Can you work these out from the model? Positions are in its coordinate system, mm. Face numbers are marked on the shaded views. A direction names the side the tool comes from. Give positions to 0.01 mm unless a question says otherwise; leave off trailing zeros. Order: outer loops, then holes, each group sorted by start corner. A loop starts at its lowest first (then second) coordinate and runs counter-clockwise, first axis right, second up. Notation, with made-up numbers: M -25.75,45.25 L -9.75,45.25 A16 cw -9.75,74.25 Z; hole C -21.5,-39 d7. An arc over 180 degrees is marked long. Write each question's results on one line, items separated by ' | '.
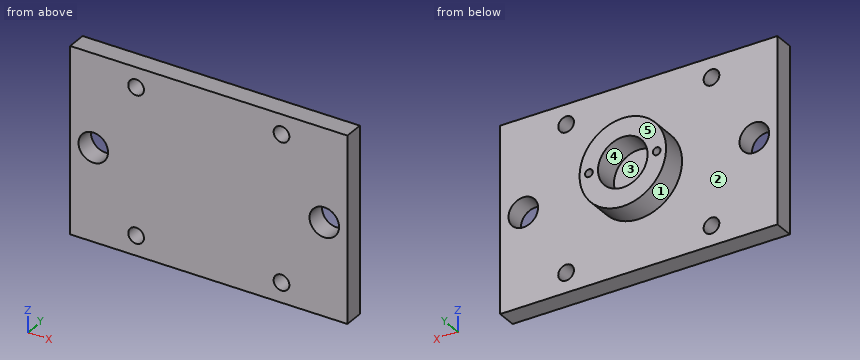
from build123d import *

# Parameters (mm, degrees)
SKETCH1_W           = 90
SKETCH1_H           = 60
SKETCH1_R           = 4.8
SKETCH1_R_2         = 2.55
BOSS_EXTRUDE1_DEPTH = 6.35
SKETCH2_R           = 14.05
SKETCH2_R_2         = 8.05
BOSS_EXTRUDE2_DEPTH = 8.175
SKETCH3_R           = 1.25
CUT_EXTRUDE1_DEPTH  = 8


with BuildPart() as part:
    # Sketch1 → Boss-Extrude1 (new body)
    with BuildSketch(Plane(origin=(0, 0, 0), x_dir=(1, 0, 0), z_dir=(0, 1, 0))):
        Rectangle(SKETCH1_W, SKETCH1_H)
        with Locations((-37.5, 0)):
            Circle(SKETCH1_R, mode=Mode.SUBTRACT)
        with Locations((37.5, 0)):
            Circle(SKETCH1_R, mode=Mode.SUBTRACT)
        with Locations((-23.6, -23.6)):
            Circle(SKETCH1_R_2, mode=Mode.SUBTRACT)
        with Locations((23.6, -23.6)):
            Circle(SKETCH1_R_2, mode=Mode.SUBTRACT)
        with Locations((23.6, 23.6)):
            Circle(SKETCH1_R_2, mode=Mode.SUBTRACT)
        with Locations((-23.6, 23.6)):
            Circle(SKETCH1_R_2, mode=Mode.SUBTRACT)
    extrude(amount=BOSS_EXTRUDE1_DEPTH)

    # Sketch2 → Boss-Extrude2 (add)
    with BuildSketch(Plane(origin=(0, 6.35, 0), x_dir=(1, 0, 0), z_dir=(0, 1, 0))):
        Circle(SKETCH2_R)
        Circle(SKETCH2_R_2, mode=Mode.SUBTRACT)
    extrude(amount=BOSS_EXTRUDE2_DEPTH)

    # Sketch3 → Cut-Extrude1 (cut)
    with BuildSketch(Plane(origin=(0, 14.525, 0), x_dir=(1, 0, 0), z_dir=(0, 1, 0))):
        with Locations((-11, 0)):
            Circle(SKETCH3_R)
        with Locations((11, 0)):
            Circle(SKETCH3_R)
    extrude(amount=-CUT_EXTRUDE1_DEPTH, mode=Mode.SUBTRACT)


solid = part.part
(1) We'd pull the mould along Z, two halves only. Please class the marked faces 1, 2 and 3: +Z half, -Z half, draft (parallel to the pull), parting line (faces both ways), or undercut.
Data:
face 1: parting line | face 2: draft | face 3: undercut
(2) Imagine slicing it at D-D, the plane x = -37.5. Write out the boundary of the cut face in (y, z), plus the area to 3 significant figures.
Data:
outline: M 0,-30 L 6.35,-30 L 6.35,-4.8 L 0,-4.8 Z; M 0,4.8 L 6.35,4.8 L 6.35,30 L 0,30 Z | area: 320 mm2
(3) I need wall thicknesses on L1, parallel to Z at x = -23.6, y = 5; L2, parallel to X at y = 1.5, z = 0; L3, parallel to X at y = 4.5, z = -23.6. Which ranges of each line are inside material? Lowest first, please. Write a range as from..to.
Data:
L1: z = -30..-26.15, -21.05..21.05, 26.15..30 | L2: x = -45..-42.3, -32.7..32.7, 42.3..45 | L3: x = -45..-26.15, -21.05..21.05, 26.15..45
(4) Imagine slicing it at B-B, the plane y = 1. Write out the boundary of the cut face in (x, z).
Data:
outline: M -45,-30 L 45,-30 L 45,30 L -45,30 Z; hole C -37.5,0 d9.6; hole C -23.6,-23.6 d5.1; hole C -23.6,23.6 d5.1; hole C 23.6,-23.6 d5.1; hole C 23.6,23.6 d5.1; hole C 37.5,0 d9.6
(5) For the marked faces 4 and 5, which set-ups out of +Z, -Z, +X, -X, +Y, -Y let a thin tool reach every point of the face, with its end or its side?
Data:
face 4: +Y | face 5: +Z, -Z, +X, -X, +Y
(6) Will these pins go through, and if not, where does the flat tip stop? P1, Ø3, axis at x = 11.5, z = 0.5, coming from the +Y side (3 decimals); P2, Ø6, axis at x = 23.6, z = -23.6, coming from the +Y side.
Data:
P1: stops at y = 14.525 | P2: stops at y = 6.35
(7) Imagine slicing it at A-A, the plane z = 0. Write out the boundary of the cut face in (x, y) (3 decimals), plus the area to 3 significant figures.
Data:
outline: M -45,0 L -42.3,0 L -42.3,6.35 L -45,6.35 Z; M -32.7,0 L 32.7,0 L 32.7,6.35 L 14.05,6.35 L 14.05,14.525 L 12.25,14.525 L 12.25,6.525 L 9.75,6.525 L 9.75,14.525 L 8.05,14.525 L 8.05,6.35 L -8.05,6.35 L -8.05,14.525 L -9.75,14.525 L -9.75,6.525 L -12.25,6.525 L -12.25,14.525 L -14.05,14.525 L -14.05,6.35 L -32.7,6.35 Z; M 42.3,0 L 45,0 L 45,6.35 L 42.3,6.35 Z | area: 508 mm2
(8) Imagine slicing it at C-C, the plane x = 23.6. Write out the boundary of the cut face in (y, z).
Data:
outline: M 0,-30 L 6.35,-30 L 6.35,-26.15 L 0,-26.15 Z; M 0,-21.05 L 6.35,-21.05 L 6.35,21.05 L 0,21.05 Z; M 0,26.15 L 6.35,26.15 L 6.35,30 L 0,30 Z
